The listing builds one solid part. Answer for the finished solid, in the listing's coordinates (mm). A direction names the side the tool comes from. Give positions to 0.01 mm unless a question says otherwise; leave off trailing zeros. Loops run counter-clockwise (first coordinate to the right, second up) from the corner with the lowest first, then second, coordinate; pieces in that order, holes last.
Item 1: Consider line 1 along X through (y, z) = (0.3, 0.55); line 2 along X through (y, z) = (0.2, -0.7); line 3 along X through (y, z) = (0.35, -0.2). Determine where each line is inside the solid, lowest interval first.
Item 2: A tool of negligible diameter and unlimited length cuts with its end or side. For faces 1 (the face through (1.3, 0.2, 0)), 2 (the face through (0, 0.5, -1)), from which of +Z, -Z, +X, -X, +Y, -Y can it reach the whole face along a straight path? Write none if from no direction.
Item 3: Section C-C, the plane x = 0.75 is taken. Give the vertices of the cut face in (y, z), and give its area (3 significant figures).
Item 4: Section B-B, the plane y = 0.25 is taken. Give the vertices of the cut face in (x, z), and give its area (3 significant figures).
Item 5: The mould has two halves that part along X. Classify faces 3 (the face through (0, 0, -1)), 4 (the face through (2, 0.2, 0)), 5 (the face through (-2.177, 0.246, 1.565)), 6 (the face through (1.6, 0.2, 0)): pulls with the +X half, pulls with the -X half, needs draft (parallel to the pull), parting line crosses it, or undercut.
Item 6: Section D-D, the plane x = -3 is taken. Give the vertices of the cut face in (y, z), and give its area (3 significant figures).
Item 7: Section A-A, the plane z = 0 is taken. Give the number of separate pieces and of enclosed holes in the cut face, and give its area (3 significant figures).
from build123d import *

# Parameters (mm, degrees)
SKETCH1_R           = 0.32069999999999993
SKETCH1_W           = 0.49999999999999956
SKETCH1_H           = 1.6
SKETCH1_R_2         = 0.3207000000000001
BOSS_EXTRUDE1_DEPTH = 0.5
FILLET3_R           = 0.15


with BuildPart() as part:
    # Sketch1 → Boss-Extrude1 (new body)
    # profile 1 of 2: a face of its own
    with BuildSketch(Plane(origin=(0, 0, 0), x_dir=(1, 0, 0), z_dir=(0, 1, 0))):
        with BuildLine():
            ThreePointArc((0.16410089999999872, 1.9932563547231181), (0.02454856527933624, 1.9949735752626254), (-0.11388375906019726, 1.9772452208459481))
            Line((-0.11388375906019724, 1.9772452208459481), (-1.2499999999996807, 1.7502411741825006))
            Line((-1.2499999999996807, 1.7502411741825006), (-1.2499999999996807, 1.2499999999996991))
            ThreePointArc((-1.2499999999996807, 1.2499999999996991), (-0.3661165235167134, 0.8838834764829733), (1.221e-14, 6.11e-15))
            ThreePointArc((1.221e-14, 5.8e-15), (-0.36611652351671364, -0.8838834764829614), (-1.249999999999681, -1.2499999999996867))
            Line((-1.2499999999996807, -1.249999999999687), (-1.2499999999996805, -1.7502411741825006))
            Line((-1.2499999999996805, -1.7502411741825006), (-0.11388375997143456, -1.9772452206638764))
            ThreePointArc((-0.11388375997143454, -1.9772452206638764), (0.02454856391169549, -1.9949735750542663), (0.16410089817752455, -1.9932563546160664))
            ThreePointArc((0.16410089817752457, -1.9932563546160669), (2.0000000001183995, -7.8577381e-10), (0.16410089999999872, 1.9932563547231181))
        make_face()
        with Locations(Location((0.5, 0, 0), (0, 0, 270))):
            Circle(SKETCH1_R, mode=Mode.SUBTRACT)
        with BuildLine():
            Line((-1.058207e-11, 1.3000000001285459), (-1.058197e-11, 1.6000000001285462))
            ThreePointArc((-1.058197e-11, 1.6000000001285457), (1.5999999999894177, 1.2854606e-10), (-1.058164e-11, -1.599999999871454))
            Line((-1.058197e-11, -1.599999999871454), (-1.058207e-11, -1.299999999871454))
            ThreePointArc((-1.058171e-11, -1.299999999871454), (1.2999999999894176, 1.2854607e-10), (-1.058207e-11, 1.3000000001285457))
        make_face(mode=Mode.SUBTRACT)
    # profile 2 of 2: a face of its own
    with BuildSketch(Plane(origin=(0, 0, 0), x_dir=(1, 0, 0), z_dir=(0, 1, 0))):
        with BuildLine():
            Line((-1.2499999999996807, 1.2499999999996991), (-1.2499999999996807, 1.7502411741825006))
            Line((-1.2499999999996807, 1.7502411741825006), (-4.1832356905240005, 1.1641599726532808))
            ThreePointArc((-4.1832356905240005, 1.1641599726532808), (-4.514100230865791, 1.0335329749029736), (-4.778306419676481, 0.7953526936222303))
            ThreePointArc((-4.778306419676481, 0.7953526936222305), (-5.05, -4.7e-16), (-4.778306419676481, -0.7953526936222314))
            ThreePointArc((-4.778306419676481, -0.7953526936222312), (-4.514100230865791, -1.033532974902974), (-4.1832356905240005, -1.1641599726532812))
            Line((-4.1832356905240005, -1.164159972653281), (-1.2499999999996805, -1.7502411741825006))
            Line((-1.2499999999996805, -1.7502411741825006), (-1.2499999999996807, -1.249999999999687))
            ThreePointArc((-1.249999999999681, -1.2499999999996867), (-2.499999999999374, 6.26e-15), (-1.2499999999996807, 1.2499999999996991))
        make_face()
        with Locations((-4, 0)):
            Rectangle(SKETCH1_W, SKETCH1_H, mode=Mode.SUBTRACT)
        with Locations(Location((-3, 0, 0), (0, 0, 270))):
            Circle(SKETCH1_R_2, mode=Mode.SUBTRACT)
    extrude(amount=BOSS_EXTRUDE1_DEPTH)

    # Fillet3
    fillet3_edges = [part.edges().sort_by_distance(p)[0] for p in [
        (-1.2499999999996816, 0, 1.2499999999996865),
        (-1.2499999999996807, 0.5, 1.249999999999687),
    ]]
    fillet(fillet3_edges, radius=FILLET3_R)


solid = part.part
Worked answers:
1. line 1: x = -4.93 to -4.25, -3.75 to -2.37, -0.13 to 1.18, 1.5 to 1.92
1. line 2: x = -4.85 to -4.25, -3.75 to -2.29, -0.21 to 1.1, 1.44 to 1.87
1. line 3: x = -5.03 to -4.25, -3.75 to -3.25, -2.75 to -2.48, -0.02 to 0.25, 0.75 to 1.28, 1.59 to 1.99
2. face 1: +Y, -Y
2. face 2: +Z, -Z, +X, -X, +Y
3. outline: (0, -1.85) - (0.5, -1.85) - (0.5, -1.41) - (0, -1.41) - close; (0, -1.06) - (0.5, -1.06) - (0.5, -0.2) - (0, -0.2) - close; (0, 0.2) - (0.5, 0.2) - (0.5, 1.06) - (0, 1.06) - close; (0, 1.41) - (0.5, 1.41) - (0.5, 1.85) - (0, 1.85) - close
3. area: 1.30 mm2
4. outline: (-4.78, -0.8) arc R1 ccw to (-4.18, -1.16) - (-0.11, -1.98) arc R1 ccw to (0.16, -1.99) arc R2 ccw to (0.16, 1.99) arc R1 ccw to (-0.11, 1.98) - (-4.18, 1.16) arc R1 ccw to (-4.78, 0.8) arc R1.3 ccw to start; hole (-4.25, -0.8) - (-3.75, -0.8) - (-3.75, 0.8) - (-4.25, 0.8) - close; hole circle Ø0.64 at (-3, 0); hole circle Ø2.5 at (-1.25, 0); hole (0, -1.6) arc R1.6 ccw to (0, 1.6) - (0, 1.3) arc R1.3 cw to (0, -1.3) - close; hole circle Ø0.64 at (0.5, 0)
4. area: 13.3 mm2
5. face 3: needs draft
5. face 4: pulls with the +X half
5. face 5: pulls with the -X half
5. face 6: undercut
6. outline: (0, -1.4) - (0.5, -1.4) - (0.5, -0.32) - (0, -0.32) - close; (0, 0.32) - (0.5, 0.32) - (0.5, 1.4) - (0, 1.4) - close
6. area: 1.08 mm2
7. separate pieces: 6
7. enclosed holes: 0
7. area: 1.21 mm2
